```python
from build123d import *

# Parameters (mm, degrees)
SKETCH_1_R                 = 2
EXTRUDE_3_DEPTH            = 2
CROQUIS1_R                 = 3.3
CROQUIS1_R_2               = 2
SALIENTE_EXTRUIR1_DEPTH    = 2.68
SKETCH_5_R                 = 2.5
EXTRUDE_7_DEPTH            = 1
CROQUIS2_R                 = 1.25
CORTAR_EXTRUIR1_DEPTH      = 4.68
CORTAR_EXTRUIR1_DEPTH_BACK = 2
CROQUIS3_R                 = 2.35
CORTAR_EXTRUIR2_DEPTH      = 1


with BuildPart() as part:
    # Эскиз1 → Бобышка-Вытянуть3 (new body)
    with BuildSketch(Plane.XY):
        with BuildLine():
            Line((-2.118749631, 2.53), (-12.106546701, 1.997159934))
            ThreePointArc((-12.106546701, 1.997159934), (-14, 0), (-12.106546701, -1.997159934))
            Line((-12.106546701, -1.997159934), (-2.118749631, -2.53))
            ThreePointArc((-2.118749631, -2.53), (0, -3.3), (2.118749631, -2.53))
            Line((2.118749631, -2.53), (12.106546701, -1.997159934))
            ThreePointArc((12.106546701, -1.997159934), (14, 0), (12.106546701, 1.997159934))
            Line((12.106546701, 1.997159934), (2.118749631, 2.53))
            ThreePointArc((2.118749631, 2.53), (0, 3.3), (-2.118749631, 2.53))
        make_face()
        Circle(SKETCH_1_R, mode=Mode.SUBTRACT)
    extrude(amount=EXTRUDE_3_DEPTH)

    # Croquis1 → Saliente-Extruir1 (add)
    with BuildSketch(Plane.XY.offset(2)):
        Circle(CROQUIS1_R)
        Circle(CROQUIS1_R_2, mode=Mode.SUBTRACT)
    extrude(amount=SALIENTE_EXTRUIR1_DEPTH)

    # Эскиз5 → Бобышка-Вытянуть7 (add)
    with BuildSketch(Plane(origin=(0, 0, 0), x_dir=(-1, 0, 0), z_dir=(0, 0, -1))):
        Circle(SKETCH_5_R)
    extrude(amount=-EXTRUDE_7_DEPTH)

    # Croquis2 → Cortar-Extruir1 (cut, two sides)
    with BuildSketch(Plane.XY.offset(1)) as cortar_extruir1_sk:
        Circle(CROQUIS2_R)
    extrude(amount=CORTAR_EXTRUIR1_DEPTH, mode=Mode.SUBTRACT)
    extrude(cortar_extruir1_sk.sketch, amount=-CORTAR_EXTRUIR1_DEPTH_BACK, mode=Mode.SUBTRACT)

    # Croquis3 → Cortar-Extruir2 (cut)
    with BuildSketch(Plane(origin=(0, 0, 0), x_dir=(-1, 0, 0), z_dir=(0, 0, -1))):
        Circle(CROQUIS3_R)
    extrude(amount=-CORTAR_EXTRUIR2_DEPTH, mode=Mode.SUBTRACT)


solid = part.part
```
The model under review builds one solid part; all positions refer to its coordinate system, in mm. A direction names the side the tool comes from. Round coordinates to 2 decimals unless told otherwise and drop trailing zeros. Loops run counter-clockwise (first coordinate to the right, second up) from the corner with the lowest first, then second, coordinate; pieces in that order, holes last. Notation, with made-up numbers: (87, 71.25) -> (92, 71.25) arc R28 cw to (92, 99.25) -> close; hole circle Ø9 at (84, 49). An arc over 180 degrees is marked (long way). Answer as a JSON object with one key per item and string values. Group by question number.
1) We need section C-C on z = 0.45. Write out the cut boundary in (x, y).
2) For faces 1 (the face through (0.509, -2.294, 0.493)), 2 (the face through (-7.18, -2.26, 0.99)), list the 3-axis set-ups (+Z, -Z, +X, -X, +Y, -Y) from which the entire face can be reached by the end or side of a thin tool; tool diameter is ignored.
3) We need section A-A on x = 0. Write out the cut boundary in (y, z), then the cut area to 3 significant figures.
4) For line 1 (Y direction, x = 0, z = 2.85); line 2 (Y direction, x = 0, z = 0.2), list the stretches that pass through material, from the lowest coordinate up. Write a range as [from, to].
5) Mouldability with a two-part tool opening along Y and no side actions: class faces 3 (the face through (7.043, -2.267, 0.986)), 4 (the face through (-14, 0, 1)), 5 (the face through (8, 0, 2)), 6 (the face through (0, -2, 3)) as released by +Y, released by -Y, zero draft, split by the parting line, or undercut.
6) We need section D-D on x = -3. Write out the cut boundary in (y, z), then the cut area to 3 significant figures.
7) We need section B-B on y = 0. Write out the cut boundary in (x, z).
8) For pin 1 Ø2.5 at (x, y) = (-5.5, 1.5) entering from +Z; pin 2 Ø2 at (y, z) = (-2, 2) entering from -X, all flat-tipped, find the tip position at first contact; note any pin that passes through.
Result set:
{
 "1": {"outline": "(-12.11, -2) -> (-2.12, -2.53) arc R3.3 ccw to (2.12, -2.53) -> (12.11, -2) arc R2 ccw to (12.11, 2) -> (2.12, 2.53) arc R3.3 ccw to (-2.12, 2.53) -> (-12.11, 2) arc R2 ccw to start; hole circle Ø4.7 at (0, 0)"},
 "2": {"face 1": "-Z", "face 2": "+Z, -Z, -X, -Y"},
 "3": {"outline": "(-3.3, 0) -> (-2.35, 0) -> (-2.35, 1) -> (-2, 1) -> (-2, 4.68) -> (-3.3, 4.68) -> close; (2, 1) -> (2.35, 1) -> (2.35, 0) -> (3.3, 0) -> (3.3, 4.68) -> (2, 4.68) -> close", "area": "11.5 mm²"},
 "4": {"line 1": "[-3.3, -2], [2, 3.3]", "line 2": "[-3.3, -2.35], [2.35, 3.3]"},
 "5": {"face 3": "released by -Y", "face 4": "split by the parting line", "face 5": "zero draft", "face 6": "undercut"},
 "6": {"outline": "(-2.48, 0) -> (2.48, 0) -> (2.48, 2) -> (1.37, 2) -> (1.37, 4.68) -> (-1.37, 4.68) -> (-1.37, 2) -> (-2.48, 2) -> close", "area": "17.3 mm²"},
 "7": {"outline": "(-14, 0) -> (-2.35, 0) -> (-2.35, 1) -> (-2, 1) -> (-2, 4.68) -> (-3.3, 4.68) -> (-3.3, 2) -> (-14, 2) -> close; (2, 1) -> (2.35, 1) -> (2.35, 0) -> (14, 0) -> (14, 2) -> (3.3, 2) -> (3.3, 4.68) -> (2, 4.68) -> close"},
 "8": {"pin 1": "z = 2", "pin 2": "x = -13.73"}
}
